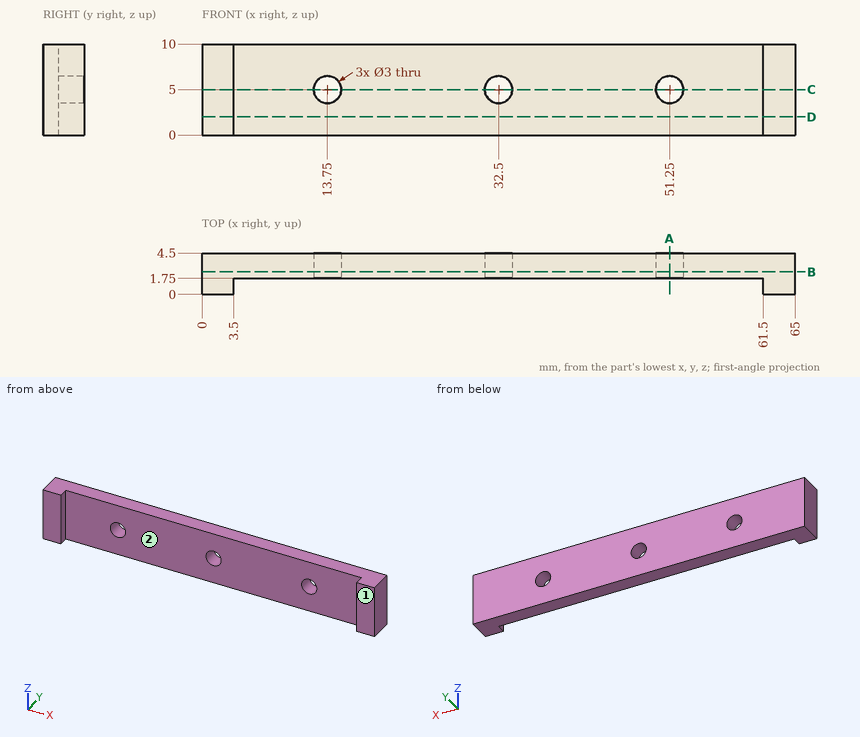
The figure shows three views and two pictorial views of one solid part (mm, origin at its lowest corner). Answer the questions. A direction names the side the tool comes from. Give positions to 0.01 mm unless a question says otherwise; leave off trailing zeros. Order: outer loops, then holes, each group sorted by start corner. A loop starts at its lowest first (then second) coordinate and runs counter-clockwise, first axis right, second up. Notation, with made-up numbers: (36.25, 73.25) -> (68.25, 73.25) arc R18 ccw to (68.25, 84.25) -> close; hole circle Ø4 at (29, 84). An arc over 180 degrees is marked (long way). Write each question's results on one line, items separated by ' | '.
Q1. The part is cut by section A-A, the plane x = 51.25. Give the vertices of the cut face in (y, z), and give its area (4 significant figures).
Checked values:
outline: (1.75, 0) -> (4.5, 0) -> (4.5, 3.5) -> (1.75, 3.5) -> close; (1.75, 6.5) -> (4.5, 6.5) -> (4.5, 10) -> (1.75, 10) -> close | area: 19.25 mm^2
Q2. The part is cut by section D-D, the plane z = 2. Give the vertices of the cut face in (x, y), and give its area (3 significant figures).
Checked values:
outline: (0, 0) -> (3.5, 0) -> (3.5, 1.75) -> (61.5, 1.75) -> (61.5, 0) -> (65, 0) -> (65, 4.5) -> (0, 4.5) -> close | area: 191 mm^2
Q3. Straight lines are drawn through the part: probe 1 along X at (y, z) = (3.1, 5); probe 2 along X at (y, z) = (0.75, 7); probe 3 along X at (y, z) = (2.2, 5.5). For each, find the intervals that lie inside material, in ascending order. Write a range as from..to.
Checked values:
probe 1: x = 0..12.25, 15.25..31, 34..49.75, 52.75..65 | probe 2: x = 0..3.5, 61.5..65 | probe 3: x = 0..12.34, 15.16..31.09, 33.91..49.84, 52.66..65
Q4. Which of the six approach directions +Z, -Z, +X, -X, +Y, -Y give full straight-line access (tool end or side, diameter ignored) to the marked faces 1 and 2?
Checked values:
face 1: +Z, -Z, +X, -X, -Y | face 2: +Z, -Z, -Y
Q5. The part is cut by section B-B, the plane y = 2.45. Give the vertices of the cut face in (x, z), and give its area (3 significant figures).
Checked values:
outline: (0, 0) -> (65, 0) -> (65, 10) -> (0, 10) -> close; hole circle Ø3 at (13.75, 5); hole circle Ø3 at (32.5, 5); hole circle Ø3 at (51.25, 5) | area: 629 mm^2
Q6. The part is cut by section C-C, the plane z = 5. Give the vertices of the cut face in (x, y).
Checked values:
outline: (0, 0) -> (3.5, 0) -> (3.5, 1.75) -> (12.25, 1.75) -> (12.25, 4.5) -> (0, 4.5) -> close; (15.25, 1.75) -> (31, 1.75) -> (31, 4.5) -> (15.25, 4.5) -> close; (34, 1.75) -> (49.75, 1.75) -> (49.75, 4.5) -> (34, 4.5) -> close; (52.75, 1.75) -> (61.5, 1.75) -> (61.5, 0) -> (65, 0) -> (65, 4.5) -> (52.75, 4.5) -> close
Q7. This flat-tipped pin is pushed along its axis until it touches: P1, Ø3, axis at x = 46.5, z = 5.5, coming from the -Y side. Where does it stop, or does it pass through?
Checked values:
P1: stops at y = 1.75
